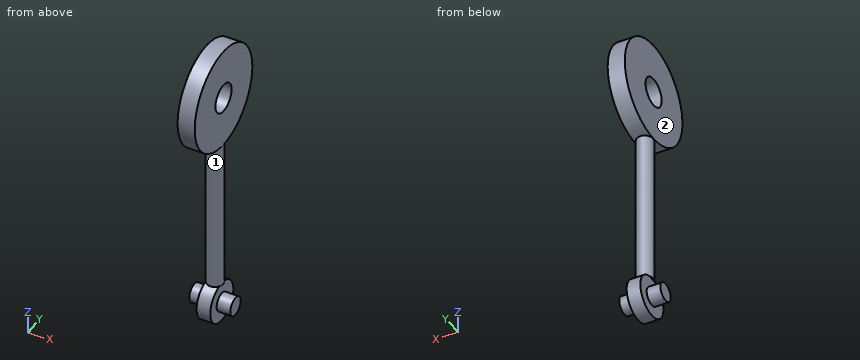
```python
from build123d import *

# Parameters (mm, degrees)
F0_R          = 9.525
F0_R_2        = 2.667
F1_DEPTH      = 1.5875
F3_START      = -5.08
F2_R          = 1.5259148542
F3_DEPTH      = 33.02
F4_R          = 3.81
F5_DEPTH      = 1.27
F6_R          = 1.7164061496
F7_DEPTH      = 2.54
F7_DEPTH_BACK = 5.08


with BuildPart() as f1:
    # F0 (on Right) → F1 (new body, symmetric)
    with BuildSketch(Plane.YZ):
        Circle(F0_R)
        Circle(F0_R_2, mode=Mode.SUBTRACT)
    extrude(amount=F1_DEPTH, both=True)

    # F2 (on Top) → F3 (join)
    with BuildSketch(Plane.XY.offset(F3_START)):
        Circle(F2_R)
    extrude(amount=-F3_DEPTH)

    # F4 (on Right) → F5 (join, symmetric)
    with BuildSketch(Plane.YZ):
        with Locations((0, -41.7686875335)):
            Circle(F4_R)
    extrude(amount=F5_DEPTH, both=True)

    # F6 (on face) → F7 (join, two sides)
    with BuildSketch(Plane(origin=(-1.27, 0, 0), x_dir=(0, -1, 0), z_dir=(-1, 0, 0))) as f7_sk:
        with Locations((0, -41.7686875335)):
            Circle(F6_R)
    extrude(amount=F7_DEPTH)
    extrude(f7_sk.sketch, amount=-F7_DEPTH_BACK)


solid = f1.part
```
Work out the finished part from the listing and answer in its coordinate system (mm). Face numbers are marked on the shaded views. Round coordinates to 2 decimals unless told otherwise and drop trailing zeros. Write each loop counter-clockwise with the first axis right and the second up, starting at its lowest first coordinate (ties: lowest second). Pieces come first, ordered by that corner, then holes.
1) Determine the mould class of the marked faces 1 and 2 for opening direction Z: pulls with the +Z half, pulls with the -Z half, needs draft (parallel to the pull), parting line crosses it, or undercut.
2) A cutting plane is placed at D-D on y = 3.25. Determine the outline of the cut face in (x, z), and give its area (3 significant figures).
3) Consider probe 1 along Z at (x, y) = (-0.25, 0) (3 decimals); probe 2 along X at (y, z) = (-2.5, -41); probe 3 along Y at (x, z) = (2.75, -41). Determine where each line is inside the solid, lowest interval first.
4) A cutting plane is placed at C-C on x = 0. Determine the outline of the cut face in (y, z) (3 decimals).
5) A cutting plane is placed at A-A on z = 0. Determine the outline of the cut face in (x, y) (1 decimal).
6) Flat-ended cylindrical pins translate along their axes: P1, Ø9.5, axis at y = -1.5, z = -2, coming from the +X side; P2, Ø1.5, axis at x = 1, z = -21, coming from the -Y side; P3, Ø6, axis at y = -2.5, z = -22, coming from the +X side. Find the tip coordinate at first contact, or state that the pin passes through.
Entries:
1. face 1: undercut
1. face 2: needs draft
2. outline: (-1.59, -8.95) - (1.59, -8.95) - (1.59, 8.95) - (-1.59, 8.95) - close; (-1.27, -43.76) - (1.27, -43.76) - (1.27, -39.78) - (-1.27, -39.78) - close
2. area: 67.0 mm2
3. probe 1: z = -45.579 to -2.667, 2.667 to 9.525
3. probe 2: x = -1.27 to 1.27
3. probe 3: y = -1.53 to 1.53
4. outline: (-1.526, -38.1) - (-1.028, -38.1) arc R3.81 ccw (long way) to (1.028, -38.1) - (1.526, -38.1) - (1.526, -9.402) arc R9.525 ccw (long way) to (-1.526, -9.402) - close; hole circle Ø5.334 at (0, 0)
5. outline: (-1.6, -9.5) - (1.6, -9.5) - (1.6, -2.7) - (-1.6, -2.7) - close; (-1.6, 2.7) - (1.6, 2.7) - (1.6, 9.5) - (-1.6, 9.5) - close
6. P1: stops at x = 1.59
6. P2: stops at y = -1.51
6. P3: stops at x = 1.53
